from build123d import *

# Parameters (mm, degrees)
F0_W     = 29
F0_H     = 42
F1_DEPTH = 29
F3_DEPTH = 12
F4_R     = 14.5
F5_DEPTH = 41


# Not quite as in the source:
# - the program builds the solid bodies; features that only make, move or delete a surface that nothing else refers to are left out


with BuildPart() as f1:
    # F0 (on Top) → F1 (new body)
    with BuildSketch(Plane.XY):
        Rectangle(F0_W, F0_H)
    extrude(amount=F1_DEPTH)

    # F2 (on face) → F3 (join)
    with BuildSketch(Plane.XZ.offset(21)):
        with BuildLine():
            ThreePointArc((0, 0), (10.2530483272, 4.2469516728), (14.5, 14.5))
            ThreePointArc((14.5, 14.5), (10.2530483272, 24.7530483272), (0, 29))
            ThreePointArc((0, 29), (-10.2530483272, 24.7530483272), (-14.5, 14.5))
            ThreePointArc((-14.5, 14.5), (-10.2530483272, 4.2469516728), (0, 0))
        make_face()
    extrude(amount=F3_DEPTH)

    # F4 (on face) → F5 (join)
    with BuildSketch(Plane.XZ.offset(33)):
        with Locations((0, 14.5)):
            Circle(F4_R)
    extrude(amount=F5_DEPTH)


solid = f1.part
Model file for the job. Use its own axes, mm. A direction names the side the tool comes from. Coordinates: 2 decimals unless noted, no trailing zeros. Order: outer loops, then holes, each group sorted by start corner. A loop starts at its lowest first (then second) coordinate and runs counter-clockwise, first axis right, second up. Notation, with made-up numbers: (-28.5, -24) -> (-9.5, -24) arc R15 ccw to (-9.5, 4) -> close; hole circle Ø1 at (21, 49). An arc over 180 degrees is marked (long way). Return JSON: item names as keys, results as strings. Group by question number.
Item 1: Saw through at B-B on z = 11. Write the cut outline in (x, y), then the cut area to 3 significant figures.
Item 2: Saw through at A-A on x = 10.5. Write the cut outline in (y, z), then the cut area to 3 significant figures.
Item 3: Tool access for faces 1 (the flat face through (11, -21, 3)), 2 (the flat face through (12, -21, 26)), 3 (the flat face through (-12, -21, 25)), 4 (the flat face through (-12, -21, 3)), 5 (the flat face through (0, 21, 14)): list every direction of +Z, -Z, +X, -X, +Y, -Y with a clear straight run to the whole face (end or side of a thin tool).
Item 4: Saw through at C-C on y = -41. Write the cut outline in (x, z), then the cut area to 3 significant figures.
Item 5: Wall check: line 1 along Y through (x, z) = (12.25, 27.5); line 2 along Z through (x, y) = (1.75, -38.5); line 3 along X through (y, z) = (-29.5, 5). Give the ranges that are in metal, low to high. Write a range as [from, to].
Item 6: Flat gauge pin, fed straight in: P1, Ø4, axis at y = -31.5, z = 14, coming from the -X side. Where does the tip first touch, or does it go through?
Values found:
{
 "1": {"outline": "(-14.5, -21) -> (-14.07, -21) -> (-14.07, -74) -> (14.07, -74) -> (14.07, -21) -> (14.5, -21) -> (14.5, 21) -> (-14.5, 21) -> close", "area": "2,710 mm2"},
 "2": {"outline": "(-74, 4.5) -> (-21, 4.5) -> (-21, 0) -> (21, 0) -> (21, 29) -> (-21, 29) -> (-21, 24.5) -> (-74, 24.5) -> close", "area": "2,280 mm2"},
 "3": {"face 1": "-Z, +X, -Y", "face 2": "+Z, +X, -Y", "face 3": "+Z, -X, -Y", "face 4": "-Z, -X, -Y", "face 5": "+Z, -Z, +X, -X, +Y"},
 "4": {"outline": "circle Ø29 at (0, 14.5)", "area": "661 mm2"},
 "5": {"line 1": "y = [-21, 21]", "line 2": "z = [0.11, 28.89]", "line 3": "x = [-10.95, 10.95]"},
 "6": {"P1": "stops at x = -14.5"}
}
